Design review of the part built by this model. Coordinates are the model's own, in mm. Face numbers are marked on the shaded views. Coordinates: 2 decimals unless noted, no trailing zeros. Order: outer loops, then holes, each group sorted by start corner. A loop starts at its lowest first (then second) coordinate and runs counter-clockwise, first axis right, second up. Notation, with made-up numbers: (45.5, -18.5) - (82.5, -18.5) arc R21 ccw to (82.5, -2.5) - close; hole circle Ø10 at (56.5, -30). An arc over 180 degrees is marked (long way). Write each question's results on one line, items separated by ' | '. Start each with the question number.
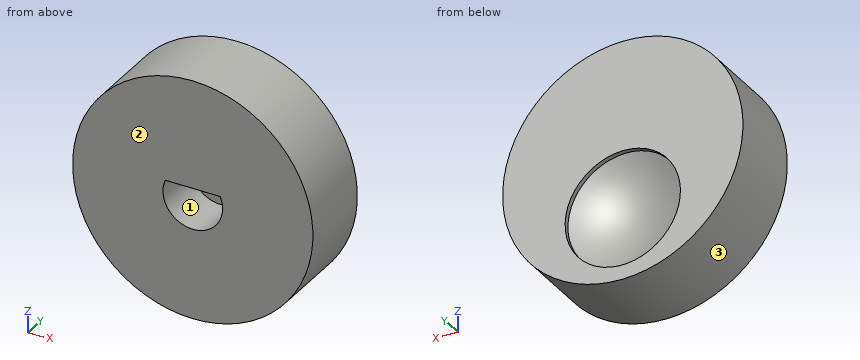
```python
from build123d import *

# Parameters (mm, degrees)
SKETCH1_R           = 12.5
BOSS_EXTRUDE1_DEPTH = 8
BOSS_EXTRUDE2_START = -3
SKETCH2_R           = 12.5
BOSS_EXTRUDE2_DEPTH = 3
SKETCH3_R           = 6
CUT_EXTRUDE1_DEPTH  = 0.5
DOME1_FACE_RADIUS   = 6
DOME1_HEIGHT        = 2


with BuildPart() as part:
    # Sketch1 → Boss-Extrude1 (new body)
    with BuildSketch(Plane(origin=(0, 0, 0), x_dir=(1, 0, 0), z_dir=(0, 1, 0))):
        with Locations(Location((0, 0, 0), (0, 0, 270))):
            Circle(SKETCH1_R)
        with BuildLine():
            Line((-2.858321186, -1.2), (2.858321186, -1.2))
            ThreePointArc((2.858321186, -1.2), (0, 3.1), (-2.858321186, -1.2))
        make_face(mode=Mode.SUBTRACT)
    extrude(amount=BOSS_EXTRUDE1_DEPTH)

    # Sketch2 → Boss-Extrude2 (add)
    with BuildSketch(Plane(origin=(0, 8, 0), x_dir=(1, 0, 0), z_dir=(0, 1, 0)).offset(BOSS_EXTRUDE2_START)):
        with Locations(Location((0, 0, 0), (0, 0, 270))):
            Circle(SKETCH2_R)
    extrude(amount=BOSS_EXTRUDE2_DEPTH)

    # Sketch3 → Cut-Extrude1 (cut)
    with BuildSketch(Plane(origin=(0, 8, 0), x_dir=(1, 0, 0), z_dir=(0, 1, 0))):
        with Locations(Location((0, 5, 0), (0, 0, 270))):
            Circle(SKETCH3_R)
    extrude(amount=-CUT_EXTRUDE1_DEPTH, mode=Mode.SUBTRACT)

    # Dome1: a dome of height H over a round flat face of radius A is a cap of a sphere of radius (A * A + H * H) / (2 * H)
    dome1_r = (DOME1_FACE_RADIUS * DOME1_FACE_RADIUS + DOME1_HEIGHT * DOME1_HEIGHT) / (2 * DOME1_HEIGHT)
    dome1_base = Plane((0, 7.5, -5), z_dir=(0, -1, 0))
    with Locations(dome1_base.offset(DOME1_HEIGHT - dome1_r)):
        dome1_ball = Sphere(dome1_r, mode=Mode.PRIVATE)
    add(split(dome1_ball, bisect_by=dome1_base, keep=Keep.TOP, mode=Mode.PRIVATE), mode=Mode.SUBTRACT)


solid = part.part
```
(1) Mouldability with a two-part tool opening along X and no side actions: class the marked faces 1, 2 and 3 as +X half, -X half, draft (parallel to the pull), parting line (faces both ways), or undercut.
(2) Take a section at D-D (x = -2.5). State the section outline as (y, z) points.
(3) Clearance check with flat-ended pins moving along their axes: pin 1 (1 mm diameter, centred on y = 4.5, z = 4.5, fed in from +X); pin 2 (2 mm diameter, centred on x = 5.5, y = 4.5, fed in from +Z); pin 3 (2 mm diameter, centred on y = 5.5, z = 3, fed in from -X). State where each tip first meets the part, or that it passes through.
(4) Take a section at C-C (z = -4). State the section outline as (x, y) points.
(5) Take a section at A-A (x = 0). State the section outline as (y, z) points.
(6) Take a section at B-B (y = 1.5). State the section outline as (x, z) points.
(7) To check wall thickness, follow line 1 along X through (y, z) = (1.25, 0); line 2 along Z through (x, y) = (-1.5, 4); line 3 along X through (y, z) = (4.5, -2.75). State the ranges of each line that lie inside material, in increasing order. Write a range as [from, to].
Worked out:
1) face 1: undercut | face 2: draft | face 3: parting line
2) outline: (0, -12.25) - (8, -12.25) - (8, -10.45) - (7.5, -10.45) arc R9.68 cw to (7.5, 0.45) - (8, 0.45) - (8, 12.25) - (0, 12.25) - (0, 1.2) - (5, 1.2) - (5, -1.83) - (0, -1.83) - close
3) pin 1: x = 11.84 | pin 2: z = 11.66 | pin 3: x = -12.34
4) outline: (-11.84, 0) - (11.84, 0) - (11.84, 8) - (5.92, 8) - (5.92, 7.5) arc R9.95 cw to (-5.92, 7.5) - (-5.92, 8) - (-11.84, 8) - close
5) outline: (0, -12.5) - (8, -12.5) - (8, -11) - (7.5, -11) arc R10 cw to (7.5, 1) - (8, 1) - (8, 12.5) - (0, 12.5) - (0, 1.2) - (5, 1.2) - (5, -3.1) - (0, -3.1) - close
6) outline: circle Ø25 at (0, 0); hole (-2.86, 1.2) arc R3.1 ccw (long way) to (2.86, 1.2) - close
7) line 1: [-12.5, -3.1], [3.1, 12.5] | line 2: [-12.41, -2.71], [1.2, 12.41] | line 3: [-12.19, -1.43], [1.43, 12.19]
